Part model, mm, in its own coordinate system. A direction names the side the tool comes from. Give positions to 0.01 mm unless a question says otherwise; leave off trailing zeros. Order: outer loops, then holes, each group sorted by start corner. A loop starts at its lowest first (then second) coordinate and runs counter-clockwise, first axis right, second up. Notation, with made-up numbers: M -33.75,6 L -3.75,6 A10 ccw -3.75,12 Z; hole C 13,13 d1. An arc over 180 degrees is marked long. Answer as a JSON object with one key per item and string values.
from build123d import *

# Parameters (mm, degrees)
BOSS_EXTRUDE1_DEPTH     = 19.05
SKETCH2_W               = 31.75
SKETCH2_H               = 6.35
BOSS_EXTRUDE2_DEPTH     = 50.8
CUT_EXTRUDE1_DEPTH      = 106.498403893
CUT_EXTRUDE1_DEPTH_BACK = 106.498403893
SKETCH3_R               = 3.175
SKETCH4_R               = 3.556
CUT_EXTRUDE2_DEPTH      = 50.8


with BuildPart() as part:
    # Sketch1 → Boss-Extrude1 (new body)
    with BuildSketch(Plane.XY):
        Polygon((0, 0), (76.2, 0), (76.2, -6.35), (12.7, -6.35), (12.7, -21.082), (76.2, -21.082), (76.2, -27.432), (0, -27.432), align=None)
    extrude(amount=BOSS_EXTRUDE1_DEPTH)

    # Sketch2 → Boss-Extrude2 (add)
    with BuildSketch(Plane.XY.offset(19.05)):
        with Locations((60.325, -24.257)):
            Rectangle(SKETCH2_W, SKETCH2_H)
    extrude(amount=BOSS_EXTRUDE2_DEPTH)

    # Sketch3 → Cut-Extrude1 (cut, two sides: drawn at the far end of the back side and taken through both)
    with BuildSketch(Plane(origin=(0, -21.082, 0), x_dir=(1, 0, 0), z_dir=(0, 1, 0)).offset(-CUT_EXTRUDE1_DEPTH_BACK)):
        with Locations(Location((63.5, -60.96, 0), (0, 0, 270))):
            Circle(SKETCH3_R)
        with Locations(Location((63.5, -9.525, 0), (0, 0, 270))):
            Circle(SKETCH3_R)
    extrude(amount=CUT_EXTRUDE1_DEPTH + CUT_EXTRUDE1_DEPTH_BACK, mode=Mode.SUBTRACT)

    # Sketch4 → Cut-Extrude2 (cut)
    with BuildSketch(Plane.ZY):
        with Locations((9.525, -13.716)):
            Circle(SKETCH4_R)
    extrude(amount=-CUT_EXTRUDE2_DEPTH, mode=Mode.SUBTRACT)


solid = part.part
1. Which spindle directions (+Z, -Z, +X, -X, +Y, -Y) get a long thin tool onto all of the face, cutting with end or side? Do faces 1 (the flat face through (46, -27.432, 27)), 2 (the flat face through (12.7, -10, 12)), 3 (the flat face through (44.45, -24, 44)), 4 (the flat face through (39, -23, 0)), 5 (the flat face through (30, -4, 19.05)). Say none if no direction does.
Worked answers:
{"face 1": "+Z, -Z, +X, -X, -Y", "face 2": "+Z, -Z, +X", "face 3": "+Z, -X, +Y, -Y", "face 4": "-Z, +X, -X, +Y, -Y", "face 5": "+Z, -X, +Y"}
2. Cut at B-B on z = 60.96. Give the cut face in (x, y) (3 decimals), plus the area to 3 significant figures.
Worked answers:
{"outline": "M 44.45,-27.432 L 60.325,-27.432 L 60.325,-21.082 L 44.45,-21.082 Z; M 66.675,-27.432 L 76.2,-27.432 L 76.2,-21.082 L 66.675,-21.082 Z", "area": "161 mm^2"}
3. Cut at C-C on y = -4. Give the cut face in (x, z) (3 decimals), plus the area to 3 significant figures.
Worked answers:
{"outline": "M 0,0 L 76.2,0 L 76.2,19.05 L 0,19.05 Z; hole C 63.5,9.525 d6.35", "area": "1,420 mm^2"}
4. Cut at A-A on x = 68.5. Give the cut face in (y, z), plus the area to 3 significant figures.
Worked answers:
{"outline": "M -27.43,0 L -21.08,0 L -21.08,69.85 L -27.43,69.85 Z; M -6.35,0 L 0,0 L 0,19.05 L -6.35,19.05 Z", "area": "565 mm^2"}
5. Probe line 1 along Z through (x, y) = (63.5, -24) (3 decimals); line 2 along Y through (x, z) = (71.5, 14); line 3 along Z through (x, y) = (63.5, -1.75). List the from-to ranges inside material, lowest first.
Worked answers:
{"line 1": "z = 0 to 6.35, 12.7 to 57.785, 64.135 to 69.85", "line 2": "y = -27.43 to -21.08, -6.35 to 0", "line 3": "z = 0 to 6.35, 12.7 to 19.05"}
6. Cut at D-D on z = 14. Give the cut face in (x, y).
Worked answers:
{"outline": "M 0,-27.43 L 76.2,-27.43 L 76.2,-21.08 L 12.7,-21.08 L 12.7,-6.35 L 76.2,-6.35 L 76.2,0 L 0,0 Z"}
7. Two-plate mould, pull along Y, no slides. Class faces 6 (the flat face through (45, -6.35, 9)), 7 (the flat face through (38, 0, 9)), 8 (the flat face through (76.2, -24, 34)): +Y half, -Y half, draft (parallel to the pull), parting line (faces both ways), or undercut.
Worked answers:
{"face 6": "undercut", "face 7": "+Y half", "face 8": "draft"}
8. Pin check, flat tips, straight feed: P1, Ø10, axis at x = 18, y = -23.5, coming from the +Z side; P2, Ø5, axis at y = -23.5, z = 41, coming from the -X side; P3, Ø10, axis at x = 63.5, z = 60.96, coming from the +Y side. Stop position of each tip, or through.
Worked answers:
{"P1": "stops at z = 19.05", "P2": "stops at x = 44.45", "P3": "stops at y = -21.08"}
